Build history of the part. All positions in model axes, mm. A direction names the side the tool comes from. Give positions to 0.01 mm unless a question says otherwise; leave off trailing zeros. Order: outer loops, then holes, each group sorted by start corner. A loop starts at its lowest first (then second) coordinate and runs counter-clockwise, first axis right, second up. Notation, with made-up numbers: (-10, -11) - (34, -11) arc R14 ccw to (34, 14) - close; hole circle Ø6 at (26, 57). An arc over 180 degrees is marked (long way). Use a Markdown table: item, result.
from build123d import *

# Parameters (mm, degrees)
MAINFRAME_DEPTH             = 11
GUIDEBACKBOARD_DEPTH        = 1
SKETCH3_W                   = 32
SKETCH3_H                   = 12
LOWELENGTH_DEPTH            = 80
SKETCH4_R                   = 8
LOWERCUT_BEARING_HOLE_DEPTH = 6
SKETCH6_R                   = 6
LOWER_BEARING_HOLE1_DEPTH   = 0.5
SKETCH7_R                   = 13
LOWER_BEARING_HOLE_2_DEPTH  = 1
SKETCH11_W                  = 55
SKETCH11_H                  = 5
BOSS_EXTRUDE1_DEPTH         = 10
BOSS_EXTRUDE1_DEPTH_BACK    = 12
SKETCH12_R                  = 2.5
CUT_EXTRUDE5_DEPTH          = 6
SKETCH13_R                  = 4
BOSS_EXTRUDE2_DEPTH         = 5


with BuildPart() as part:
    # Sketch1 → MainFrame (new body)
    with BuildSketch(Plane.XY):
        Polygon((-16, 61.475378035), (16, 61.475378035), (16, 0), (10, 0), (10, 55.475378035), (-10, 55.475378035), (-10, 0), (-16, 0), align=None)
    extrude(amount=MAINFRAME_DEPTH)

    # Sketch2 → GuideBackBoard (add)
    with BuildSketch(Plane(origin=(0, 0, 0), x_dir=(-1, 0, 0), z_dir=(0, 0, -1))):
        Polygon((8, 0), (8, 55.975378035), (-8, 55.975378035), (-8, 0), (-16, 0), (-16, 61.475378035), (16, 61.475378035), (16, 0), align=None)
    extrude(amount=GUIDEBACKBOARD_DEPTH)

    # Sketch3 → LoweLength (add)
    with BuildSketch(Plane.XZ):
        with Locations((0, 5)):
            Rectangle(SKETCH3_W, SKETCH3_H)
    extrude(amount=LOWELENGTH_DEPTH)

    # Sketch4 → LowerCut Bearing Hole (cut)
    with BuildSketch(Plane.XY.offset(11)):
        with Locations((0, -42.024621965)):
            Circle(SKETCH4_R)
    extrude(amount=-LOWERCUT_BEARING_HOLE_DEPTH, mode=Mode.SUBTRACT)

    # Sketch6 → Lower Bearing Hole1 (cut)
    with BuildSketch(Plane.XY.offset(5)):
        with Locations((0, -42.024621965)):
            Circle(SKETCH6_R)
    extrude(amount=-LOWER_BEARING_HOLE1_DEPTH, mode=Mode.SUBTRACT)

    # Sketch7 → Lower Bearing Hole 2 (cut)
    with BuildSketch(Plane.XY.offset(11)):
        with Locations((0, -42.024621965)):
            Circle(SKETCH7_R)
    extrude(amount=-LOWER_BEARING_HOLE_2_DEPTH, mode=Mode.SUBTRACT)

    # Sketch11 → Boss-Extrude1 (add, two sides)
    with BuildSketch(Plane.XY.offset(11)) as boss_extrude1_sk:
        with Locations((0, -77.5)):
            Rectangle(SKETCH11_W, SKETCH11_H)
    extrude(amount=BOSS_EXTRUDE1_DEPTH)
    extrude(boss_extrude1_sk.sketch, amount=-BOSS_EXTRUDE1_DEPTH_BACK)

    # Sketch12 → Cut-Extrude5 (cut, through all)
    with BuildSketch(Plane(origin=(0, -75, 0), x_dir=(1, 0, 0), z_dir=(0, 1, 0))):
        with Locations((21, -4)):
            Circle(SKETCH12_R)
        with Locations((-21, -4)):
            Circle(SKETCH12_R)
    extrude(amount=-CUT_EXTRUDE5_DEPTH, mode=Mode.SUBTRACT)

    # Sketch13 → Boss-Extrude2 (add)
    with BuildSketch(Plane.XZ.offset(-55.475378035)):
        with Locations((0, 5.5)):
            Circle(SKETCH13_R)
    extrude(amount=BOSS_EXTRUDE2_DEPTH)


solid = part.part
1) Tool access for faces 1 (the flat face through (0, 50.475, 6)), 2 (the cylindrical face through (-0.867, 53.01, 1.595)), 3 (the flat face through (0, 0, 5)), 4 (the flat face through (0, -6, 11)), 5 (the flat face through (16, -6, 5)): list every direction of +Z, -Z, +X, -X, +Y, -Y with a clear straight run to the whole face (end or side of a thin tool).
Computed:
| item | result |
|---|---|
| face 1 | +Z, -Z |
| face 2 | none |
| face 3 | +Z |
| face 4 | +Z, +X, -X, +Y |
| face 5 | +Z, -Z, +X, +Y |
2) Slice it at D-D (x = 0). Write the cut outline in (y, z), and give its area (3 significant figures).
Computed:
| item | result |
|---|---|
| outline | (-80, -1) - (0, -1) - (0, 11) - (-29.02, 11) - (-29.02, 10) - (-34.02, 10) - (-34.02, 5) - (-36.02, 5) - (-36.02, 4.5) - (-48.02, 4.5) - (-48.02, 5) - (-50.02, 5) - (-50.02, 10) - (-55.02, 10) - (-55.02, 11) - (-75, 11) - (-75, 21) - (-80, 21) - close; (50.48, 1.5) - (55.48, 1.5) - (55.48, 0) - (55.98, 0) - (55.98, -1) - (61.48, -1) - (61.48, 11) - (55.48, 11) - (55.48, 9.5) - (50.48, 9.5) - close |
| area | 1,010 mm² |
3) Pin check, flat tips, straight feed: P1, Ø5.5, axis at y = 33.5, z = 3.5, coming from the +X side; P2, Ø5, axis at x = 21.5, z = 17.5, coming from the +Y side; P3, Ø5, axis at x = -5, y = -1.5, coming from the +Z side; P4, Ø4, axis at x = 21, z = 4, coming from the -Y side. Stop position of each tip, or through.
Computed:
| item | result |
|---|---|
| P1 | stops at x = 16 |
| P2 | stops at y = -75 |
| P3 | stops at z = 11 |
| P4 | passes through |
4) Slice it at B-B (y = 14.5). Write the cut outline in (x, z), and give its area (3 significant figures).
Computed:
| item | result |
|---|---|
| outline | (-16, -1) - (-8, -1) - (-8, 0) - (-10, 0) - (-10, 11) - (-16, 11) - close; (8, -1) - (16, -1) - (16, 11) - (10, 11) - (10, 0) - (8, 0) - close |
| area | 148 mm² |
5) Wall check: line 1 (Y direction, x = 0, z = 4.7); line 2 (Y direction, x = 0, z = 10.6); line 3 (X direction, y = -77, z = 4). Give the ranges that are in metal, low to high. Write a range as from..to.
Computed:
| item | result |
|---|---|
| line 1 | y = -80..-48.02, -36.02..0, 50.48..61.48 |
| line 2 | y = -80..-55.02, -29.02..0, 55.48..61.48 |
| line 3 | x = -27.5..-23.5, -18.5..18.5, 23.5..27.5 |
6) Slice it at A-A (x = 21). Write the cut outline in (y, z), and give its area (3 significant figures).
Computed:
| item | result |
|---|---|
| outline | (-80, -1) - (-75, -1) - (-75, 1.5) - (-80, 1.5) - close; (-80, 6.5) - (-75, 6.5) - (-75, 21) - (-80, 21) - close |
| area | 85.0 mm² |
7) Slice it at C-C (y = -45.5). Write the cut outline in (x, z), and give its area (3 significant figures).
Computed:
| item | result |
|---|---|
| outline | (-16, -1) - (16, -1) - (16, 11) - (12.53, 11) - (12.53, 10) - (7.21, 10) - (7.21, 5) - (4.89, 5) - (4.89, 4.5) - (-4.89, 4.5) - (-4.89, 5) - (-7.21, 5) - (-7.21, 10) - (-12.53, 10) - (-12.53, 11) - (-16, 11) - close |
| area | 282 mm² |
8) Two-plate mould, pull along Z, no slides. Class faces 6 (the flat face through (0, -24, -1)), 7 (the cylindrical face through (-23.5, -77.5, 3.9)), 8 (the flat face through (-16, -6, 5)), 9 (the flat face through (-2, -36, 5)): +Z half, -Z half, draft (parallel to the pull), parting line (faces both ways), or undercut.
Computed:
| item | result |
|---|---|
| face 6 | -Z half |
| face 7 | undercut |
| face 8 | draft |
| face 9 | +Z half |
